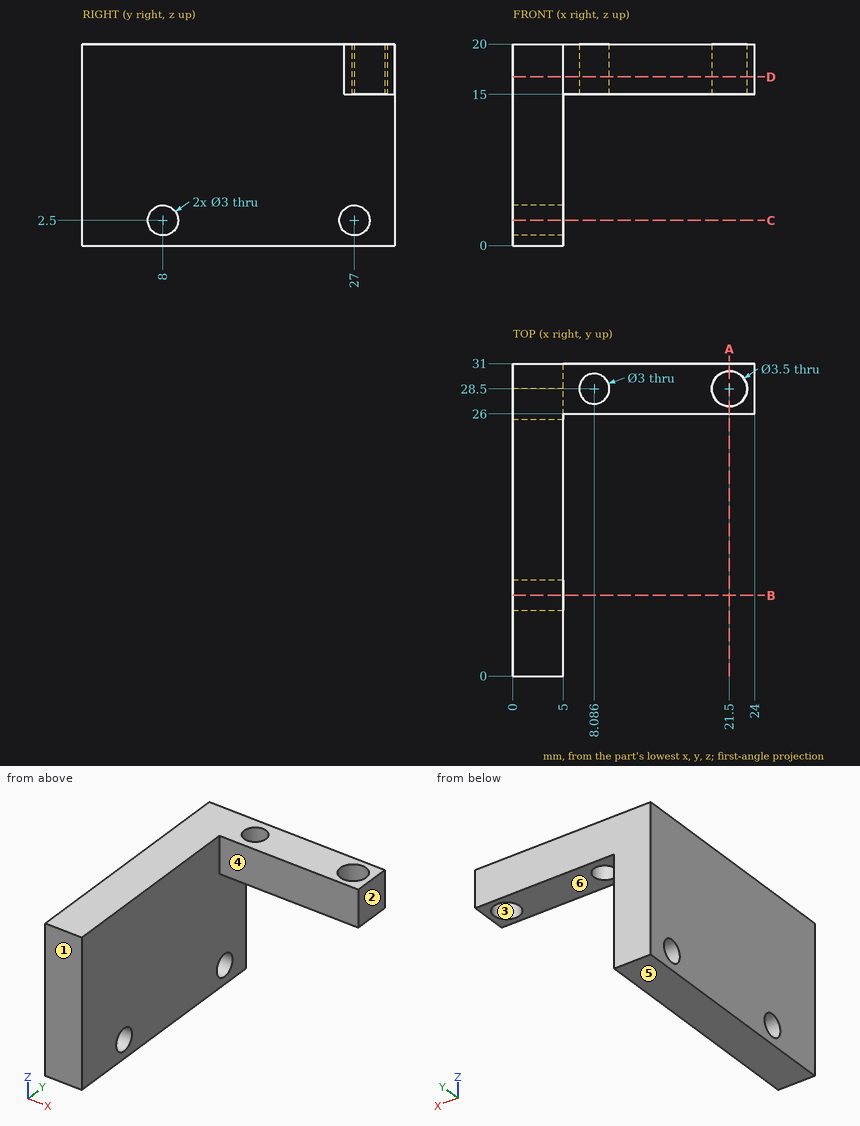
The figure shows three views and two pictorial views of one solid part (mm, origin at its lowest corner). Answer the questions. A direction names the side the tool comes from. Give positions to 0.01 mm unless a question says otherwise; leave off trailing zeros. Loops run counter-clockwise (first coordinate to the right, second up) from the corner with the lowest first, then second, coordinate; pieces in that order, holes last. Notation, with made-up numbers: (-6.5, -8.5) -> (20.5, -8.5) arc R20 cw to (20.5, 13.5) -> close; hole circle Ø4 at (29, -8.5). An arc over 180 degrees is marked (long way). Use a Markdown table: item, result. Add a question column.
1. Determine the mould class of the marked faces 1, 2 and 3 for opening direction Y: released by +Y, released by -Y, zero draft, split by the parting line, or undercut.
2. For the marked faces 4, 5 and 6, determine the directions among +Z, -Z, +X, -X, +Y, -Y from which every point of the face is accessible in a straight line to the end or side of a thin tool.
3. Section C-C on z = 2.5 is taken. Determine the outline of the cut face in (x, y).
4. Flat-ended cylindrical pins translate along their axes: pin 1 Ø4 at (x, y) = (11.5, 29) entering from -Z; pin 2 Ø10 at (y, z) = (11, 18) entering from -X; pin 3 Ø2 at (y, z) = (10.5, 17) entering from +X; pin 4 Ø2 at (x, z) = (17.5, 13) entering from -Y. Find the tip coordinate at first contact, or state that the pin passes through.
5. Find the intervals of material crossed by probe 1 along Y at (x, z) = (21.5, 18.9); probe 2 along Z at (x, y) = (8.5, 30); probe 3 along X at (y, z) = (6, 4.25), in increasing order.
6. Section A-A on x = 21.5 is taken. Determine the outline of the cut face in (y, z).
7. Section B-B on y = 8 is taken. Determine the outline of the cut face in (x, z).
8. Section D-D on z = 16.75 is taken. Determine the outline of the cut face in (x, y), and give its area (3 significant figures).
Results below:
| question | item | result |
|---|---|---|
| 1 | face 1 | released by -Y |
| 1 | face 2 | zero draft |
| 1 | face 3 | undercut |
| 2 | face 4 | +Z, -Z, +X, -Y |
| 2 | face 5 | -Z, +X, -X, +Y, -Y |
| 2 | face 6 | -Z, +X, +Y, -Y |
| 3 | outline | (0, 0) -> (5, 0) -> (5, 6.5) -> (0, 6.5) -> close; (0, 9.5) -> (5, 9.5) -> (5, 25.5) -> (0, 25.5) -> close; (0, 28.5) -> (5, 28.5) -> (5, 31) -> (0, 31) -> close |
| 4 | pin 1 | stops at z = 15 |
| 4 | pin 2 | stops at x = 0 |
| 4 | pin 3 | stops at x = 5 |
| 4 | pin 4 | passes through |
| 5 | probe 1 | y = 26 to 26.75, 30.25 to 31 |
| 5 | probe 2 | z = 15 to 20 |
| 5 | probe 3 | x = 0 to 5 |
| 6 | outline | (26, 15) -> (26.75, 15) -> (26.75, 20) -> (26, 20) -> close; (30.25, 15) -> (31, 15) -> (31, 20) -> (30.25, 20) -> close |
| 7 | outline | (0, 0) -> (5, 0) -> (5, 1) -> (0, 1) -> close; (0, 4) -> (5, 4) -> (5, 20) -> (0, 20) -> close |
| 8 | outline | (0, 0) -> (5, 0) -> (5, 26) -> (24, 26) -> (24, 31) -> (0, 31) -> close; hole circle Ø3 at (8.09, 28.5); hole circle Ø3.5 at (21.5, 28.5) |
| 8 | area | 233 mm^2 |
